```python
from build123d import *

# Parameters (mm, degrees)
SKETCH_1_R             = 6
EXTRUDE_1_DEPTH        = 10.8
CHAMFER_1_SIZE         = 1
CHAMFER_1_SIZE2        = 2.144506921
CHAMFER_1_PART_2_SIZE  = 1
CHAMFER_1_PART_2_SIZE2 = 2.144506921
CHAMFER_1_PART_3_SIZE  = 1
CHAMFER_1_PART_3_SIZE2 = 2.144506921
CHAMFER_1_PART_4_SIZE  = 1
CHAMFER_1_PART_4_SIZE2 = 2.144506921
CHAMFER_1_PART_5_SIZE  = 1
CHAMFER_1_PART_5_SIZE2 = 2.144506921
CHAMFER_1_PART_6_SIZE  = 1
CHAMFER_1_PART_6_SIZE2 = 2.144506921
CHAMFER_2_SIZE         = 1
CHAMFER_2_SIZE2        = 2.144506921
CHAMFER_2_PART_2_SIZE  = 1
CHAMFER_2_PART_2_SIZE2 = 2.144506921
CHAMFER_2_PART_3_SIZE  = 1
CHAMFER_2_PART_3_SIZE2 = 2.144506921
CHAMFER_2_PART_4_SIZE  = 1
CHAMFER_2_PART_4_SIZE2 = 2.144506921
CHAMFER_2_PART_5_SIZE  = 1
CHAMFER_2_PART_5_SIZE2 = 2.144506921
CHAMFER_2_PART_6_SIZE  = 1
CHAMFER_2_PART_6_SIZE2 = 2.144506921
FILLET_2_R             = 12


with BuildPart() as part:
    # Эскиз1 → Бобышка-Вытянуть1 (new body)
    with BuildSketch(Plane(origin=(0, 0, 0), x_dir=(1, 0, 0), z_dir=(0, 1, 0))):
        Polygon((0, 9.95), (-8.616952768, 4.975), (-8.616952768, -4.975), (0, -9.95), (8.616952768, -4.975), (8.616952768, 4.975), align=None)
        Circle(SKETCH_1_R, mode=Mode.SUBTRACT)
    extrude(amount=EXTRUDE_1_DEPTH)

    # Фаска1
    chamfer_1_edges = [part.edges().sort_by_distance(p)[0] for p in [
        (-8.616952768, 10.8, 0),
    ]]
    chamfer_1_side = [part.faces().sort_by_distance(p)[0] for p in [
        (-8.616952768, 5.4, 0),
    ]]
    chamfer(chamfer_1_edges, length=CHAMFER_1_SIZE, length2=CHAMFER_1_SIZE2, reference=chamfer_1_side[0])

    # Фаска1 part 2
    chamfer_1_part_2_edges = [part.edges().sort_by_distance(p)[0] for p in [
        (-4.308476384, 10.8, 7.4625),
    ]]
    chamfer_1_part_2_side = [part.faces().sort_by_distance(p)[0] for p in [
        (-4.308476384, 5.4, 7.4625),
    ]]
    chamfer(chamfer_1_part_2_edges, length=CHAMFER_1_PART_2_SIZE, length2=CHAMFER_1_PART_2_SIZE2, reference=chamfer_1_part_2_side[0])

    # Фаска1 part 3
    chamfer_1_part_3_edges = [part.edges().sort_by_distance(p)[0] for p in [
        (4.308476384, 10.8, 7.4625),
    ]]
    chamfer_1_part_3_side = [part.faces().sort_by_distance(p)[0] for p in [
        (4.308476384, 5.4, 7.4625),
    ]]
    chamfer(chamfer_1_part_3_edges, length=CHAMFER_1_PART_3_SIZE, length2=CHAMFER_1_PART_3_SIZE2, reference=chamfer_1_part_3_side[0])

    # Фаска1 part 4
    chamfer_1_part_4_edges = [part.edges().sort_by_distance(p)[0] for p in [
        (8.616952768, 10.8, 0),
    ]]
    chamfer_1_part_4_side = [part.faces().sort_by_distance(p)[0] for p in [
        (8.616952768, 5.4, 0),
    ]]
    chamfer(chamfer_1_part_4_edges, length=CHAMFER_1_PART_4_SIZE, length2=CHAMFER_1_PART_4_SIZE2, reference=chamfer_1_part_4_side[0])

    # Фаска1 part 5
    chamfer_1_part_5_edges = [part.edges().sort_by_distance(p)[0] for p in [
        (4.308476384, 10.8, -7.4625),
    ]]
    chamfer_1_part_5_side = [part.faces().sort_by_distance(p)[0] for p in [
        (4.308476384, 5.4, -7.4625),
    ]]
    chamfer(chamfer_1_part_5_edges, length=CHAMFER_1_PART_5_SIZE, length2=CHAMFER_1_PART_5_SIZE2, reference=chamfer_1_part_5_side[0])

    # Фаска1 part 6
    chamfer_1_part_6_edges = [part.edges().sort_by_distance(p)[0] for p in [
        (-4.308476384, 10.8, -7.4625),
    ]]
    chamfer_1_part_6_side = [part.faces().sort_by_distance(p)[0] for p in [
        (-4.308476384, 5.4, -7.4625),
    ]]
    chamfer(chamfer_1_part_6_edges, length=CHAMFER_1_PART_6_SIZE, length2=CHAMFER_1_PART_6_SIZE2, reference=chamfer_1_part_6_side[0])

    # Фаска2
    chamfer_2_edges = [part.edges().sort_by_distance(p)[0] for p in [
        (8.616952768, 0, 0),
    ]]
    chamfer_2_side = [part.faces().sort_by_distance(p)[0] for p in [
        (8.616952768, 4.9, 0),
    ]]
    chamfer(chamfer_2_edges, length=CHAMFER_2_SIZE, length2=CHAMFER_2_SIZE2, reference=chamfer_2_side[0])

    # Фаска2 part 2
    chamfer_2_part_2_edges = [part.edges().sort_by_distance(p)[0] for p in [
        (4.308476384, 0, 7.4625),
    ]]
    chamfer_2_part_2_side = [part.faces().sort_by_distance(p)[0] for p in [
        (4.308476384, 4.9, 7.4625),
    ]]
    chamfer(chamfer_2_part_2_edges, length=CHAMFER_2_PART_2_SIZE, length2=CHAMFER_2_PART_2_SIZE2, reference=chamfer_2_part_2_side[0])

    # Фаска2 part 3
    chamfer_2_part_3_edges = [part.edges().sort_by_distance(p)[0] for p in [
        (-4.308476384, 0, 7.4625),
    ]]
    chamfer_2_part_3_side = [part.faces().sort_by_distance(p)[0] for p in [
        (-4.308476384, 4.9, 7.4625),
    ]]
    chamfer(chamfer_2_part_3_edges, length=CHAMFER_2_PART_3_SIZE, length2=CHAMFER_2_PART_3_SIZE2, reference=chamfer_2_part_3_side[0])

    # Фаска2 part 4
    chamfer_2_part_4_edges = [part.edges().sort_by_distance(p)[0] for p in [
        (-8.616952768, 0, 0),
    ]]
    chamfer_2_part_4_side = [part.faces().sort_by_distance(p)[0] for p in [
        (-8.616952768, 4.9, 0),
    ]]
    chamfer(chamfer_2_part_4_edges, length=CHAMFER_2_PART_4_SIZE, length2=CHAMFER_2_PART_4_SIZE2, reference=chamfer_2_part_4_side[0])

    # Фаска2 part 5
    chamfer_2_part_5_edges = [part.edges().sort_by_distance(p)[0] for p in [
        (-4.308476384, 0, -7.4625),
    ]]
    chamfer_2_part_5_side = [part.faces().sort_by_distance(p)[0] for p in [
        (-4.308476384, 4.9, -7.4625),
    ]]
    chamfer(chamfer_2_part_5_edges, length=CHAMFER_2_PART_5_SIZE, length2=CHAMFER_2_PART_5_SIZE2, reference=chamfer_2_part_5_side[0])

    # Фаска2 part 6
    chamfer_2_part_6_edges = [part.edges().sort_by_distance(p)[0] for p in [
        (4.308476384, 0, -7.4625),
    ]]
    chamfer_2_part_6_side = [part.faces().sort_by_distance(p)[0] for p in [
        (4.308476384, 4.9, -7.4625),
    ]]
    chamfer(chamfer_2_part_6_edges, length=CHAMFER_2_PART_6_SIZE, length2=CHAMFER_2_PART_6_SIZE2, reference=chamfer_2_part_6_side[0])

    # Скругление2
    fillet_2_edges = [part.edges().sort_by_distance(p)[0] for p in [
        (7.544699307, 0.5, 4.355934176),
        (0, 0.5, 8.711868352),
        (7.544699307, 0.5, -4.355934176),
        (-7.544699307, 0.5, 4.355934176),
        (0, 0.5, -8.711868352),
        (-7.544699307, 0.5, -4.355934176),
    ]]
    fillet(fillet_2_edges, radius=FILLET_2_R)


solid = part.part
```
Geometry: final body of the model. Coordinates: model frame, mm. Round coordinates to 2 decimals unless told otherwise and drop trailing zeros. Loops run counter-clockwise (first coordinate to the right, second up) from the corner with the lowest first, then second, coordinate; pieces in that order, holes last. Notation, with made-up numbers: (68.5, 78.25) -> (87.5, 78.25) arc R8 ccw to (87.5, 87.25) -> close; hole circle Ø2 at (16, -34). An arc over 180 degrees is marked (long way). Use one line per item in the form item = value. Start each with the question number.
1) Section B-B on y = 9. Output: boundary loops of the cut face in (x, z) (3 decimals).
2) Section A-A on z = 0. Output: boundary loops of the cut face in (x, y).
3) First-contact query: P1, Ø2, axis at x = -5.5, z = 7, coming from the -Y side; P2, Ø1, axis at x = 2.5, y = 4.5, coming from the +Z side; P3, Ø1.5, axis at y = 5.5, z = 7, coming from the -X side; P4, Ø6, axis at x = 0.5, y = 4.5, coming from the -Z side. Flat tips, straight axial feed; report the tip coordinate or a pass-through.
4) Line query: L1, parallel to X at y = 8.25, z = 0; L2, parallel to Z at x = -1, y = 1; L3, parallel to Z at x = 1, y = 3.25. Output: solid intervals per line, ascending.
5) Draft query along X for faces 1 (the cylindrical face through (-0.04, 0.51, 8)), 2 (the cylindrical face through (-6.9, 0.5, 4)), 3 (the cylindrical face through (-6, 5, 0)), 4 (the flat face through (8.617, 5, 0)). Return one class per face: released by +X, released by -X, zero draft, split by the parting line, or undercut.
Response:
q1.outline = (-8.617, -4.975) -> (0, -9.95) -> (8.617, -4.975) -> (8.617, 4.975) -> (0, 9.95) -> (-8.617, 4.975) -> close; hole circle Ø12 at (0, 0)
q2.outline = (-8.62, 1) -> (-6.47, 0) -> (-6, 0) -> (-6, 10.8) -> (-6.47, 10.8) -> (-8.62, 9.8) -> close; (6, 0) -> (6.47, 0) -> (8.62, 1) -> (8.62, 9.8) -> (6.47, 10.8) -> (6, 10.8) -> close
q3.P1 = 0.62
q3.P2 = 8.8
q3.P3 = -6.41
q3.P4 = -9.95
q4.L1 = -8.62 to -6, 6 to 8.62
q4.L2 = -9.1 to -5.92, 5.92 to 9.1
q4.L3 = -9.37 to -5.92, 5.92 to 9.37
q5.face_1 = split by the parting line
q5.face_2 = released by -X
q5.face_3 = undercut
q5.face_4 = released by +X
